Part print with two shaded views. Sizes in mm from the minimum x, y, z corner. A direction names the side the tool comes from. Round coordinates to 2 decimals unless told otherwise and drop trailing zeros. Loops run counter-clockwise (first coordinate to the right, second up) from the corner with the lowest first, then second, coordinate; pieces in that order, holes last. Notation, with made-up numbers: M 62,-26.5 L 88,-26.5 A19 ccw 88,-8.5 Z; hole C 63,-1.75 d4. An arc over 180 degrees is marked long. Use a Markdown table: item, result. Add a question column.
Item 1: Saw through at B-B on y = 10.5. Write the cut outline in (x, z).
Item 2: Saw through at C-C on x = 16.5. Write the cut outline in (y, z).
Item 3: Tool access for the marked faces 4 and 5: list every direction of +Z, -Z, +X, -X, +Y, -Y with a clear straight run to the whole face (end or side of a thin tool).
Item 4: Saw through at A-A on z = 7.5. Write the cut outline in (x, y).
Item 5: Two-plate mould, pull along X, no slides. Class the marked faces 1, 2 and 3: +X half, -X half, draft (parallel to the pull), parting line (faces both ways), or undercut.
Item 6: Wall check: L1, parallel to X at y = 7.5, z = 8; L2, parallel to X at y = 2.25, z = 46.5; L3, parallel to Z at x = 25, y = 11.5. Give the ranges that are in metal, low to high. Write a range as from..to.
Item 7: Saw through at D-D on x = 30. Write the cut outline in (y, z), then the cut area to 3 significant figures.
Item 8: Pin check, flat tips, straight feed: P1, Ø2, axis at x = 8.5, y = 5.5, coming from the +Z side; P2, Ø12, axis at x = 38.5, z = 16.5, coming from the +Y side. Stop position of each tip, or through.
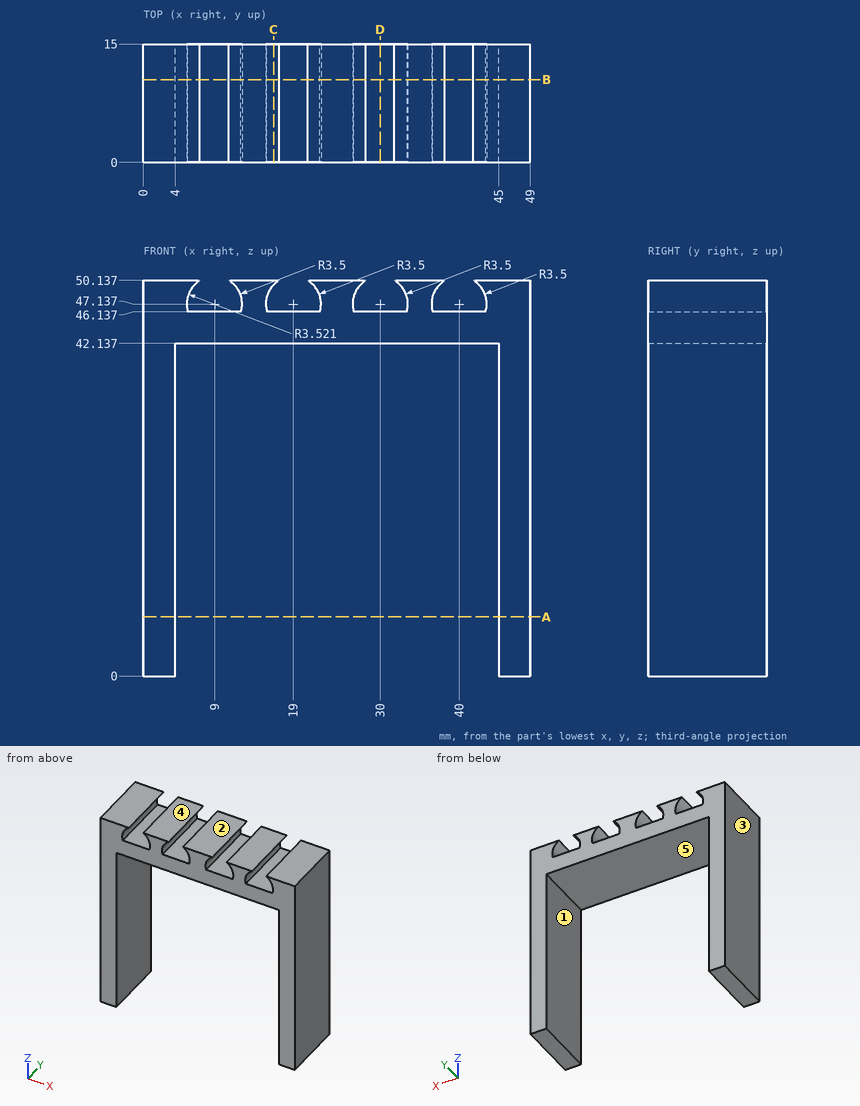
Entries:
| question | item | result |
|---|---|---|
| 1 | outline | M 0,0 L 4,0 L 4,42.14 L 45,42.14 L 45,0 L 49,0 L 49,50.14 L 41.8,50.14 A3.5 cw 43.35,46.14 L 36.65,46.14 A3.5 cw 38.2,50.14 L 31.8,50.14 A3.5 cw 33.35,46.14 L 26.65,46.14 A3.5 cw 28.2,50.14 L 20.8,50.14 A3.5 cw 22.35,46.14 L 15.65,46.14 A3.5 cw 17.2,50.14 L 10.8,50.14 A3.5 cw 12.35,46.14 L 5.62,46.14 A3.52 cw 7.16,50.14 L 0,50.14 Z |
| 2 | outline | M 0,42.14 L 15,42.14 L 15,46.14 L 0,46.14 Z; M 0,49.59 L 15,49.59 L 15,50.14 L 0,50.14 Z |
| 3 | face 4 | +Z, +X, -X, +Y, -Y |
| 3 | face 5 | -Z, +Y, -Y |
| 4 | outline | M 0,0 L 4,0 L 4,15 L 0,15 Z; M 45,0 L 49,0 L 49,15 L 45,15 Z |
| 5 | face 1 | undercut |
| 5 | face 2 | draft |
| 5 | face 3 | -X half |
| 6 | L1 | 0..4, 45..49 |
| 6 | L2 | 0..5.54, 12.44..15.56, 22.44..26.56, 33.44..36.56, 43.44..49 |
| 6 | L3 | 42.14..50.14 |
| 7 | outline | M 0,42.14 L 15,42.14 L 15,46.14 L 0,46.14 Z |
| 7 | area | 60.0 mm2 |
| 8 | P1 | z = 46.14 |
| 8 | P2 | through |
